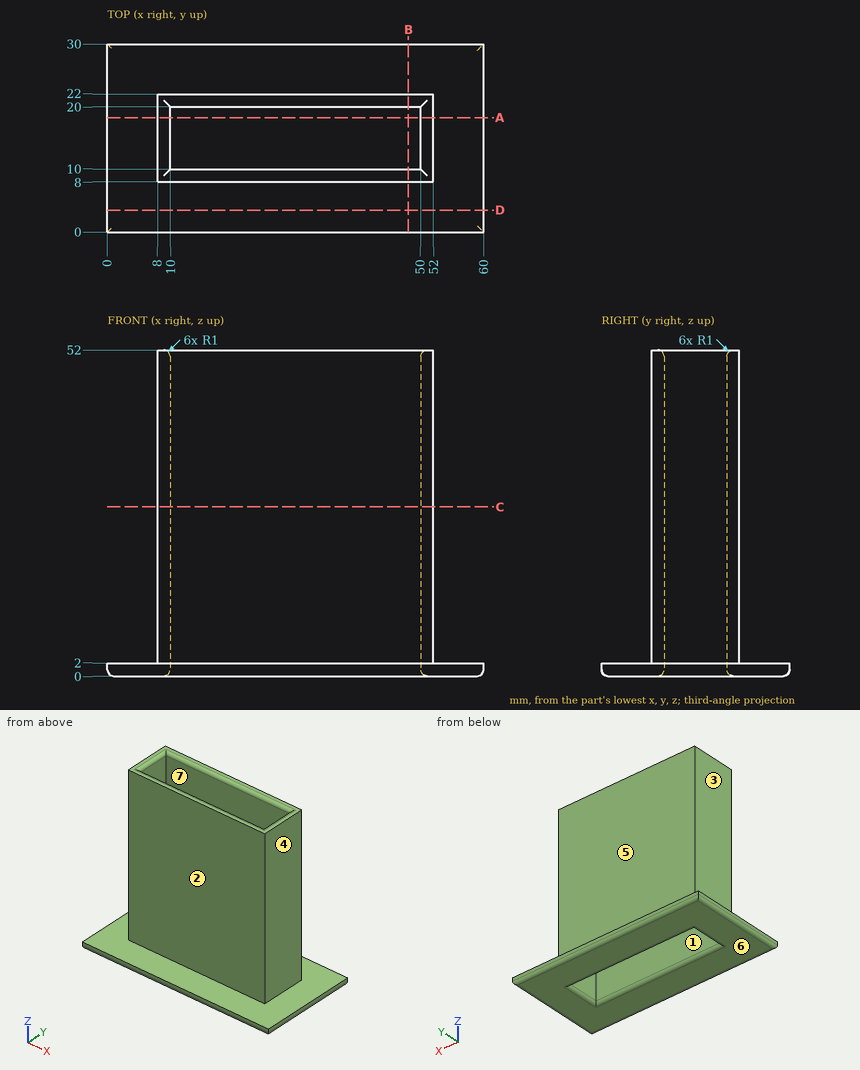
Study the drawing (mm; zero at the part's minimum x, y, z) and answer. A direction names the side the tool comes from. Coordinates: 2 decimals unless noted, no trailing zeros. Write each loop counter-clockwise with the first axis right and the second up, starting at its lowest first coordinate (ties: lowest second). Pieces come first, ordered by that corner, then holes. Notation, with made-up numbers: (21, -28) - (64, -28) arc R7 ccw to (64, -15) - close; hole circle Ø9 at (23.5, 63). An arc over 180 degrees is marked (long way). One line per question, with ' | ' between items.
1) Find section A-A, the plane y = 18.25. Determine the outline of the cut face in (x, z), and give its area (3 significant figures).
Checks:
outline: (0, 1) arc R1 ccw to (1, 0) - (9, 0) arc R1 ccw to (10, 1) - (10, 51) arc R1 ccw to (9, 52) - (8, 52) - (8, 2) - (0, 2) - close; (50, 1) arc R1 ccw to (51, 0) - (59, 0) arc R1 ccw to (60, 1) - (60, 2) - (52, 2) - (52, 52) - (51, 52) arc R1 ccw to (50, 51) - close | area: 239 mm2
2) Find section B-B, the plane x = 48. Determine the outline of the cut face in (y, z).
Checks:
outline: (0, 1) arc R1 ccw to (1, 0) - (9, 0) arc R1 ccw to (10, 1) - (10, 51) arc R1 ccw to (9, 52) - (8, 52) - (8, 2) - (0, 2) - close; (20, 1) arc R1 ccw to (21, 0) - (29, 0) arc R1 ccw to (30, 1) - (30, 2) - (22, 2) - (22, 52) - (21, 52) arc R1 ccw to (20, 51) - close
3) Find section C-C, the plane z = 27. Determine the outline of the cut face in (x, y), and give its area (3 significant figures).
Checks:
outline: (8, 8) - (52, 8) - (52, 22) - (8, 22) - close; hole (10, 10) - (50, 10) - (50, 20) - (10, 20) - close | area: 216 mm2
4) The mould has two halves that part along X. Classify the marked faces 1, 2 and 3: +X half, -X half, draft (parallel to the pull), parting line (faces both ways), or undercut.
Checks:
face 1: undercut | face 2: draft | face 3: -X half
5) Consider probe 1 along X at (y, z) = (11.5, 6); probe 2 along Y at (x, z) = (49.5, 37); probe 3 along Z at (x, y) = (28.5, 5.25). Determine where each line is inside the solid, lowest interval first. Write a range as [from, to].
Checks:
probe 1: [8, 10], [50, 52] | probe 2: [8, 10], [20, 22] | probe 3: [0, 2]
6) Find section D-D, the plane y = 3.5. Determine the outline of the cut face in (x, z), and give its area (3 significant figures).
Checks:
outline: (0, 1) arc R1 ccw to (1, 0) - (59, 0) arc R1 ccw to (60, 1) - (60, 2) - (0, 2) - close | area: 120 mm2
7) Flat-ended cylindrical pins translate along their axes: P1, Ø5, axis at y = 14, z = 19.5, coming from the -X side; P2, Ø5, axis at y = 20, z = 20, coming from the +X side; P3, Ø1, axis at x = 38, z = 46.5, coming from the +Y side; P4, Ø6, axis at y = 25.5, z = 29, coming from the -X side. Find the tip coordinate at first contact, or state that the pin passes through.
Checks:
P1: x = 8 | P2: x = 52 | P3: y = 22 | P4: through
8) For the marked faces 4, 5, 6 and 7, determine the directions among +Z, -Z, +X, -X, +Y, -Y from which every point of the face is accessible in a straight line to the end or side of a thin tool.
Checks:
face 4: +Z, +X, +Y, -Y | face 5: +Z, +X, -X, +Y | face 6: -Z, +X, -X, +Y, -Y | face 7: +Z, -Z
